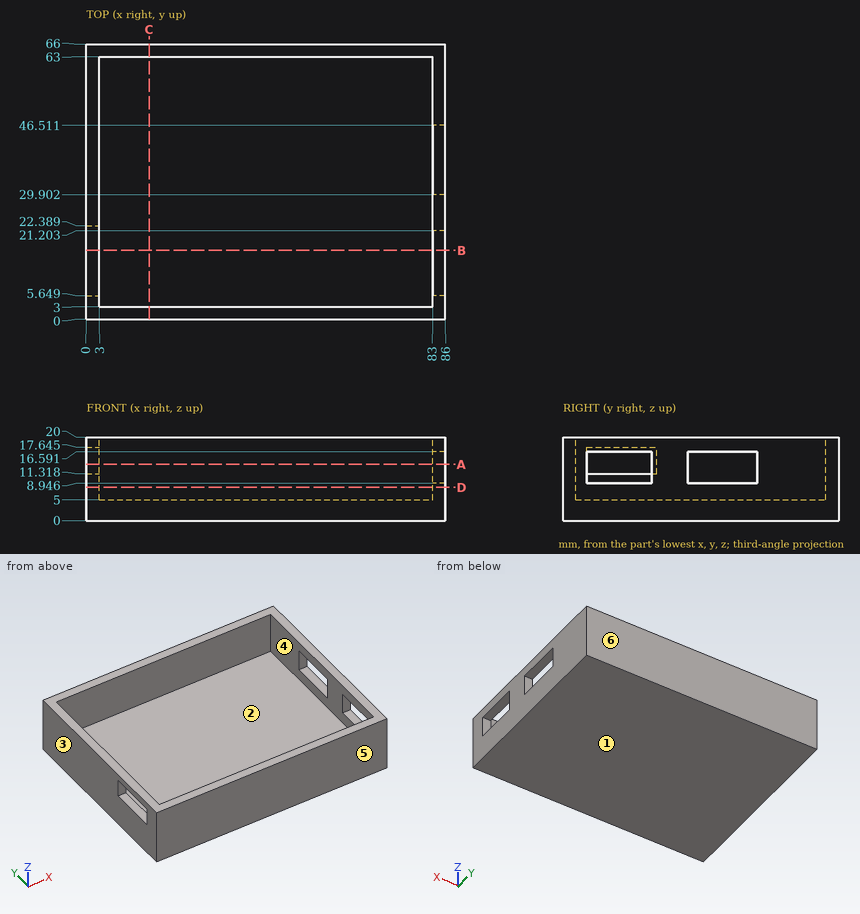
Drawing for the job (mm, zero at the part's lowest x, y, z). A direction names the side the tool comes from. Give positions to 0.01 mm unless a question says otherwise; leave off trailing zeros. Loops run counter-clockwise (first coordinate to the right, second up) from the corner with the lowest first, then second, coordinate; pieces in that order, holes last. Notation, with made-up numbers: M 25.5,69 L 83.5,69 A12 cw 83.5,79 Z; hole C 53.25,23.5 d7. An arc over 180 degrees is marked long. One line per question, with ' | ' between items. Start each with the question number.
1. Two-plate mould, pull along Y, no slides. Class the marked faces 3, 4, 5 and 6: pulls with the +Y half, pulls with the -Y half, needs draft (parallel to the pull), parting line crosses it, or undercut.
2. Saw through at C-C on x = 15. Give the cut face in (y, z).
3. Probe L1, parallel to X at y = 26.5, z = 7.5; L2, parallel to Y at x = 49, z = 6; L3, parallel to Z at x = 39.5, y = 8.5. List the from-to ranges inside material, lowest first. Write a range as from..to.
4. Saw through at A-A on z = 13.5. Give the cut face in (x, y).
5. 3-axis set-ups, long thin cutter, end or side, ignore diameter. For the marked faces 1 and 2: which of +Z, -Z, +X, -X, +Y, -Y reach the whole face in a straight line?
6. Saw through at B-B on y = 16.5. Give the cut face in (x, z) (1 decimal).
7. Flat gauge pins, fed straight in: pin 1 (6 mm diameter, centred on x = 20, y = 10.5, fed in from +Z); pin 2 (2 mm diameter, centred on y = 43.5, z = 12, fed in from +X). Where does each tip first touch, or does it go through?
8. Saw through at D-D on z = 8. Give the cut face in (x, y).
Result sheet:
1) face 3: needs draft | face 4: undercut | face 5: pulls with the -Y half | face 6: pulls with the +Y half
2) outline: M 0,0 L 66,0 L 66,20 L 63,20 L 63,5 L 3,5 L 3,20 L 0,20 Z
3) L1: x = 0..3, 83..86 | L2: y = 0..3, 63..66 | L3: z = 0..5
4) outline: M 0,0 L 86,0 L 86,5.65 L 83,5.65 L 83,3 L 3,3 L 3,5.65 L 0,5.65 Z; M 0,22.39 L 3,22.39 L 3,63 L 83,63 L 83,46.51 L 86,46.51 L 86,66 L 0,66 Z; M 83,21.2 L 86,21.2 L 86,29.9 L 83,29.9 Z
5) face 1: -Z, +X, -X, +Y, -Y | face 2: +Z
6) outline: M 0,0 L 86,0 L 86,8.9 L 83,8.9 L 83,5 L 3,5 L 3,11.3 L 0,11.3 Z; M 0,17.6 L 3,17.6 L 3,20 L 0,20 Z; M 83,16.6 L 86,16.6 L 86,20 L 83,20 Z
7) pin 1: stops at z = 5 | pin 2: stops at x = 3
8) outline: M 0,0 L 86,0 L 86,66 L 0,66 Z; hole M 3,3 L 83,3 L 83,63 L 3,63 Z
